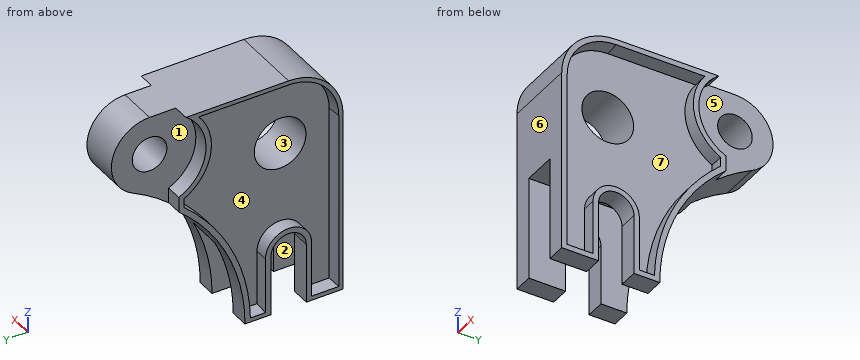
```python
from build123d import *
from OCP.BRepFilletAPI import BRepFilletAPI_MakeChamfer

# Parameters (mm, degrees)
SKETCH2_R           = 6.35
BOSS_EXTRUDE1_DEPTH = 7.25
BOSS_EXTRUDE2_DEPTH = 13.25
SKETCH2_4_R         = 9.5
BOSS_EXTRUDE3_DEPTH = 8.25
CHAMFER1_SIZE       = 0.437443318
CHAMFER1_SIZE_2     = 5
SKETCH3_W           = 12.5
SKETCH3_H           = 38
CUT_EXTRUDE1_DEPTH  = 50


with BuildPart() as part:
    # Sketch2 → Boss-Extrude1 (new, symmetric)
    with BuildSketch(Plane(origin=(0, 0, 0), x_dir=(0, 0, -1), z_dir=(1, 0, 0))):
        with BuildLine():
            ThreePointArc((-17.444074423, 30.751237722), (-33.17807799, 38.221892264), (-44.012704688, 24.584428722))
            Line((-44.012704688, 24.584428722), (-44.012704688, 14.940777961))
            ThreePointArc((-44.012704688, 14.940777961), (-43.308060102, 13.990396231), (-42.539020478, 13.091325888))
            ThreePointArc((-42.539020478, 13.091325888), (-27.32091807, 7.798890756), (-14.520771303, 17.584428722))
            Line((-14.520771303, 17.584428722), (-8.941749337, 17.584428722))
            ThreePointArc((-8.941749337, 17.584428722), (-13.579253126, 23.918357524), (-17.444074423, 30.751237722))
        make_face()
        with Locations(Location((-30.012704688, 24.584428722, 0), (0, 0, 180))):
            Circle(SKETCH2_R, mode=Mode.SUBTRACT)
    extrude(amount=BOSS_EXTRUDE1_DEPTH, both=True)

    # Sketch2<3> → Boss-Extrude2 (add, symmetric)
    with BuildSketch(Plane(origin=(0, 0, 0), x_dir=(0, 0, -1), z_dir=(1, 0, 0))):
        with BuildLine():
            ThreePointArc((-42.539020478, 13.091325888), (-43.308060102, 13.990396231), (-44.012704688, 14.940777961))
            Line((-44.012704688, 14.940777961), (-44.012704688, -22.736176348))
            ThreePointArc((-44.012704688, -22.736176348), (-38.154840312, -36.878311972), (-24.012704688, -42.736176348))
            Line((-24.012704688, -42.736176348), (42.705798991, -42.736176348))
            Line((42.705798991, -42.736176348), (42.705798991, -29.236176348))
            Line((42.705798991, -29.236176348), (20.705798991, -29.236176348))
            ThreePointArc((20.705798991, -29.236176348), (14.205798991, -22.736176348), (20.705798991, -16.236176348))
            Line((20.705798991, -16.236176348), (42.705798991, -16.236176348))
            Line((42.705798991, -16.236176348), (42.705798991, -6.736176348))
            ThreePointArc((42.705798991, -6.736176348), (14.162143482, -0.351848663), (-8.941749337, 17.584428722))
            Line((-8.941749337, 17.584428722), (-14.520771303, 17.584428722))
            ThreePointArc((-14.520771303, 17.584428722), (-27.32091807, 7.798890756), (-42.539020478, 13.091325888))
        make_face()
        with BuildLine():
            ThreePointArc((-42.012704688, 9.853508859), (-26.296300857, 5.951438018), (-13.279504157, 15.584428722))
            Line((-13.279504157, 15.584428722), (-9.875106941, 15.584428722))
            ThreePointArc((-9.875106941, 15.584428722), (12.834584681, -1.93513579), (40.705798991, -8.70718475))
            Line((40.705798991, -8.70718475), (40.705798991, -14.236176348))
            Line((40.705798991, -14.236176348), (20.705798991, -14.236176348))
            ThreePointArc((20.705798991, -14.236176348), (12.205798991, -22.736176348), (20.705798991, -31.236176348))
            Line((20.705798991, -31.236176348), (40.705798991, -31.236176348))
            Line((40.705798991, -31.236176348), (40.705798991, -40.736176348))
            Line((40.705798991, -40.736176348), (-24.012704688, -40.736176348))
            ThreePointArc((-24.012704688, -40.736176348), (-36.74062675, -35.464098409), (-42.012704688, -22.736176348))
            Line((-42.012704688, -22.736176348), (-42.012704688, 9.853508859))
        make_face(mode=Mode.SUBTRACT)
    extrude(amount=BOSS_EXTRUDE2_DEPTH, both=True)

    # Sketch2<4> → Boss-Extrude3 (add, symmetric)
    with BuildSketch(Plane(origin=(0, 0, 0), x_dir=(0, 0, -1), z_dir=(1, 0, 0))):
        with BuildLine():
            Line((-42.012704688, 9.853508859), (-42.012704688, -22.736176348))
            ThreePointArc((-42.012704688, -22.736176348), (-36.74062675, -35.464098409), (-24.012704688, -40.736176348))
            Line((-24.012704688, -40.736176348), (40.705798991, -40.736176348))
            Line((40.705798991, -40.736176348), (40.705798991, -31.236176348))
            Line((40.705798991, -31.236176348), (20.705798991, -31.236176348))
            ThreePointArc((20.705798991, -31.236176348), (12.205798991, -22.736176348), (20.705798991, -14.236176348))
            Line((20.705798991, -14.236176348), (40.705798991, -14.236176348))
            Line((40.705798991, -14.236176348), (40.705798991, -8.70718475))
            ThreePointArc((40.705798991, -8.70718475), (12.834584681, -1.93513579), (-9.875106941, 15.584428722))
            Line((-9.875106941, 15.584428722), (-13.279504157, 15.584428722))
            ThreePointArc((-13.279504157, 15.584428722), (-26.296300857, 5.951438018), (-42.012704688, 9.853508859))
        make_face()
        with Locations((-17.294201009, -22.736176348)):
            Circle(SKETCH2_4_R, mode=Mode.SUBTRACT)
    extrude(amount=BOSS_EXTRUDE3_DEPTH, both=True)

    # Chamfer1
    chamfer1_edges_1 = [part.edges().sort_by_distance(p)[0] for p in [
        (-13.25, -40.736176348, -8.346547152),
    ]]
    chamfer1_side_1 = [part.faces().sort_by_distance(p)[0] for p in [
        (-13.25, -40.744925214, -8.346547152),
    ]]
    chamfer1_edges_2 = [part.edges().sort_by_distance(p)[0] for p in [
        (-13.25, -35.464098409, 36.74062675),
    ]]
    chamfer1_side_2 = [part.faces().sort_by_distance(p)[0] for p in [
        (-13.25, -35.470284792, 36.746813132),
    ]]
    chamfer1_edges_3 = [part.edges().sort_by_distance(p)[0] for p in [
        (-13.25, -6.441333744, 42.012704688),
    ]]
    chamfer1_side_3 = [part.faces().sort_by_distance(p)[0] for p in [
        (-13.25, -6.441333744, 42.021453555),
    ]]
    chamfer1_edges_4 = [part.edges().sort_by_distance(p)[0] for p in [
        (8.25, -40.736176348, -8.346547152),
    ]]
    chamfer1_side_4 = [part.faces().sort_by_distance(p)[0] for p in [
        (8.258748866, -40.736176348, -8.346547152),
    ]]
    chamfer1_edges_5 = [part.edges().sort_by_distance(p)[0] for p in [
        (8.25, -35.464098409, 36.74062675),
    ]]
    chamfer1_side_5 = [part.faces().sort_by_distance(p)[0] for p in [
        (8.258748866, -35.464098409, 36.74062675),
    ]]
    chamfer1_edges_6 = [part.edges().sort_by_distance(p)[0] for p in [
        (8.25, -6.441333744, 42.012704688),
    ]]
    chamfer1_side_6 = [part.faces().sort_by_distance(p)[0] for p in [
        (8.258748866, -6.441333744, 42.012704688),
    ]]
    chamfer1_edges_7 = [part.edges().sort_by_distance(p)[0] for p in [
        (-13.25, -35.986176348, -40.705798991),
    ]]
    chamfer1_side_7 = [part.faces().sort_by_distance(p)[0] for p in [
        (-13.25, -35.986176348, -40.714547858),
    ]]
    chamfer1_edges_8 = [part.edges().sort_by_distance(p)[0] for p in [
        (-13.25, -11.471680549, -40.705798991),
    ]]
    chamfer1_side_8 = [part.faces().sort_by_distance(p)[0] for p in [
        (-13.25, -11.471680549, -40.714547858),
    ]]
    chamfer1_edges_9 = [part.edges().sort_by_distance(p)[0] for p in [
        (8.25, -35.986176348, -40.705798991),
    ]]
    chamfer1_side_9 = [part.faces().sort_by_distance(p)[0] for p in [
        (8.258748866, -35.986176348, -40.705798991),
    ]]
    chamfer1_edges_10 = [part.edges().sort_by_distance(p)[0] for p in [
        (8.25, -11.471680549, -40.705798991),
    ]]
    chamfer1_side_10 = [part.faces().sort_by_distance(p)[0] for p in [
        (8.258748866, -11.471680549, -40.705798991),
    ]]
    chamfer1 = BRepFilletAPI_MakeChamfer(part.part.solid().wrapped)
    for e in chamfer1_edges_1:
        chamfer1.Add(CHAMFER1_SIZE - 0.0001, CHAMFER1_SIZE_2 - 0.0001, e.wrapped, chamfer1_side_1[0].wrapped)
    for e in chamfer1_edges_2:
        chamfer1.Add(CHAMFER1_SIZE - 0.0001, CHAMFER1_SIZE_2 - 0.0001, e.wrapped, chamfer1_side_2[0].wrapped)
    for e in chamfer1_edges_3:
        chamfer1.Add(CHAMFER1_SIZE - 0.0001, CHAMFER1_SIZE_2 - 0.0001, e.wrapped, chamfer1_side_3[0].wrapped)
    for e in chamfer1_edges_4:
        chamfer1.Add(CHAMFER1_SIZE_2 - 0.0001, CHAMFER1_SIZE - 0.0001, e.wrapped, chamfer1_side_4[0].wrapped)
    for e in chamfer1_edges_5:
        chamfer1.Add(CHAMFER1_SIZE_2 - 0.0001, CHAMFER1_SIZE - 0.0001, e.wrapped, chamfer1_side_5[0].wrapped)
    for e in chamfer1_edges_6:
        chamfer1.Add(CHAMFER1_SIZE_2 - 0.0001, CHAMFER1_SIZE - 0.0001, e.wrapped, chamfer1_side_6[0].wrapped)
    for e in chamfer1_edges_7:
        chamfer1.Add(CHAMFER1_SIZE - 0.0001, CHAMFER1_SIZE_2 - 0.0001, e.wrapped, chamfer1_side_7[0].wrapped)
    for e in chamfer1_edges_8:
        chamfer1.Add(CHAMFER1_SIZE - 0.0001, CHAMFER1_SIZE_2 - 0.0001, e.wrapped, chamfer1_side_8[0].wrapped)
    for e in chamfer1_edges_9:
        chamfer1.Add(CHAMFER1_SIZE_2 - 0.0001, CHAMFER1_SIZE - 0.0001, e.wrapped, chamfer1_side_9[0].wrapped)
    for e in chamfer1_edges_10:
        chamfer1.Add(CHAMFER1_SIZE_2 - 0.0001, CHAMFER1_SIZE - 0.0001, e.wrapped, chamfer1_side_10[0].wrapped)
    add(Compound.cast(chamfer1.Shape()), mode=Mode.REPLACE)  # a hair under: the kernel refuses the full size

    # Sketch3 → Cut-Extrude1 (cut)
    with BuildSketch(Plane(origin=(0, 0, 0), x_dir=(1, 0, 0), z_dir=(0, 1, 0))):
        with Locations((0, 23.705798991)):
            Rectangle(SKETCH3_W, SKETCH3_H)
    extrude(amount=-CUT_EXTRUDE1_DEPTH, mode=Mode.SUBTRACT)


solid = part.part
```
Source: CAD feature listing. Evaluate the final solid. Frame: model axes, mm. Face numbers are marked on the shaded views. A direction names the side the tool comes from. Round coordinates to 2 decimals unless told otherwise and drop trailing zeros. Write each loop counter-clockwise with the first axis right and the second up, starting at its lowest first coordinate (ties: lowest second). Pieces come first, ordered by that corner, then holes. Notation, with made-up numbers: M -39,-31 L -31,-31 A16 cw -31,-19 Z; hole C 11,-6.5 d8. An arc over 180 degrees is marked long. Answer as a JSON object with one key per item and string values. Group by question number.
(1) First-contact query: pin 1 (9.5 mm diameter, centred on y = 25.5, z = 25, fed in from +X); pin 2 (1 mm diameter, centred on x = -7, y = 29.5, fed in from +Z); pin 3 (1.5 mm diameter, centred on x = -10, z = -23.5, fed in from +Y). Flat tips, straight axial feed; report the tip coordinate or a pass-through.
(2) Section query A-A on x = -4.25. Output: boundary loops of the cut face in (y, z).
(3) Reachability of the marked faces 1, 2, 3 and 4 from +Z, -Z, +X, -X, +Y, -Y: full face, straight path, thin tool, end or side. Return the list, or none.
(4) Ray query, line 1 (X direction, y = -33, z = -20.5); line 2 (Y direction, x = 12, z = -22.5); line 3 (X direction, y = -29.5, z = 2.5). Return the intervals inside material, ascending. Write a range as [from, to].
(5) Section query B-B on z = -32.5. State how many separate pieces and enclosed holes the cut face has, then the cut area to 3 significant figures.
(6) Section query C-C on x = -10.5. Output: boundary loops of the cut face in (y, z).
(7) Mould query, pull axis Y, two halves, no side actions, for the marked faces 5, 6 and 7. Classes: +Y half, -Y half, draft (parallel to the pull), parting line (faces both ways), or undercut.
Computed values:
{
 "1": {"pin 1": "x = 7.25", "pin 2": "z = 43.3", "pin 3": "y = -3.7"},
 "2": {"outline": "M -42.74,-4.71 L 0,-4.71 L 0,-13.43 A67 cw 30.75,17.44 A14 ccw 24.58,44.01 L -22.74,44.01 A20 ccw -42.74,24.01 Z; hole C -22.74,17.29 d19; hole C 24.58,30.01 d12.7"},
 "3": {"face 1": "-X, +Y", "face 2": "-Z, -Y", "face 3": "+X, -X", "face 4": "-X"},
 "4": {"line 1": "[-8.25, -6.25], [6.25, 8.25]", "line 2": "[-42.74, -40.63], [-31.24, -29.24], [-16.24, -14.24], [-5.71, -3.62]", "line 3": "[-8.25, 8.25]"},
 "5": {"separate pieces": "4", "enclosed holes": "0", "area": "175 mm^2"},
 "6": {"outline": "M -42.74,-42.71 L -29.24,-42.71 L -29.24,-20.71 A6.5 cw -16.24,-20.71 L -16.24,-42.71 L -6.74,-42.71 A67 cw 17.58,8.94 L 17.58,14.52 A17 cw 14.94,44.01 L -22.74,44.01 A20 ccw -42.74,24.01 Z; hole M -40.93,-40.9 L -31.24,-40.9 L -31.24,-20.71 A8.5 cw -14.24,-20.71 L -14.24,-40.9 L -8.71,-40.9 A69 cw 15.58,9.88 L 15.58,13.28 A19 cw 10.02,42.21 L -22.74,42.21 A18.2 ccw -40.93,24.01 Z"},
 "7": {"face 5": "draft", "face 6": "-Y half", "face 7": "undercut"}
}
